Design review of the part shown in the three views and the two pictorial views. Dimensions are in mm from the part's minimum x, y and z. A direction names the side the tool comes from. Coordinates: 2 decimals unless noted, no trailing zeros. Order: outer loops, then holes, each group sorted by start corner. A loop starts at its lowest first (then second) coordinate and runs counter-clockwise, first axis right, second up. Notation, with made-up numbers: (28.5, -4) - (85.5, -4) arc R15 cw to (85.5, 23) - close; hole circle Ø9 at (35.5, 69.25). An arc over 180 degrees is marked (long way). One line per item, written item: value. Start each with the question number.
(1) Mouldability with a two-part tool opening along X and no side actions: class the marked faces 1, 2 and 3 as released by +X, released by -X, zero draft, split by the parting line, or undercut.
(2) Consider section A-A on y = 35. Write out the cut boundary in (x, z).
(3) To check wall thickness, follow line 1 along X through (y, z) = (48.5, 45); line 2 along Z through (x, y) = (4.5, 8.5); line 3 along Y through (x, z) = (46.5, 34). State the ranges of each line that lie inside material, in increasing order.
(4) Consider section D-D on z = 37. Write out the cut boundary in (x, y).
(5) Consider section C-C on z = 9.5. Write out the cut boundary in (x, y).
(6) Consider section B-B on x = 71. Write out the cut boundary in (y, z), then the cut area to 3 significant figures.
(7) For the marked faces 4, 5 and 6, list the 3-axis set-ups (+Z, -Z, +X, -X, +Y, -Y) from which the entire face can be reached by the end or side of a thin tool; tool diameter is ignored.
(8) Clearance check with flat-ended pins moving along their axes: pin 1 (1.5 mm diameter, centred on x = 49.5, z = 38.5, fed in from -Y); pin 2 (12.5 mm diameter, centred on x = 64, y = 44.5, fed in from +Z). State where each tip first meets the part, or that it passes through.
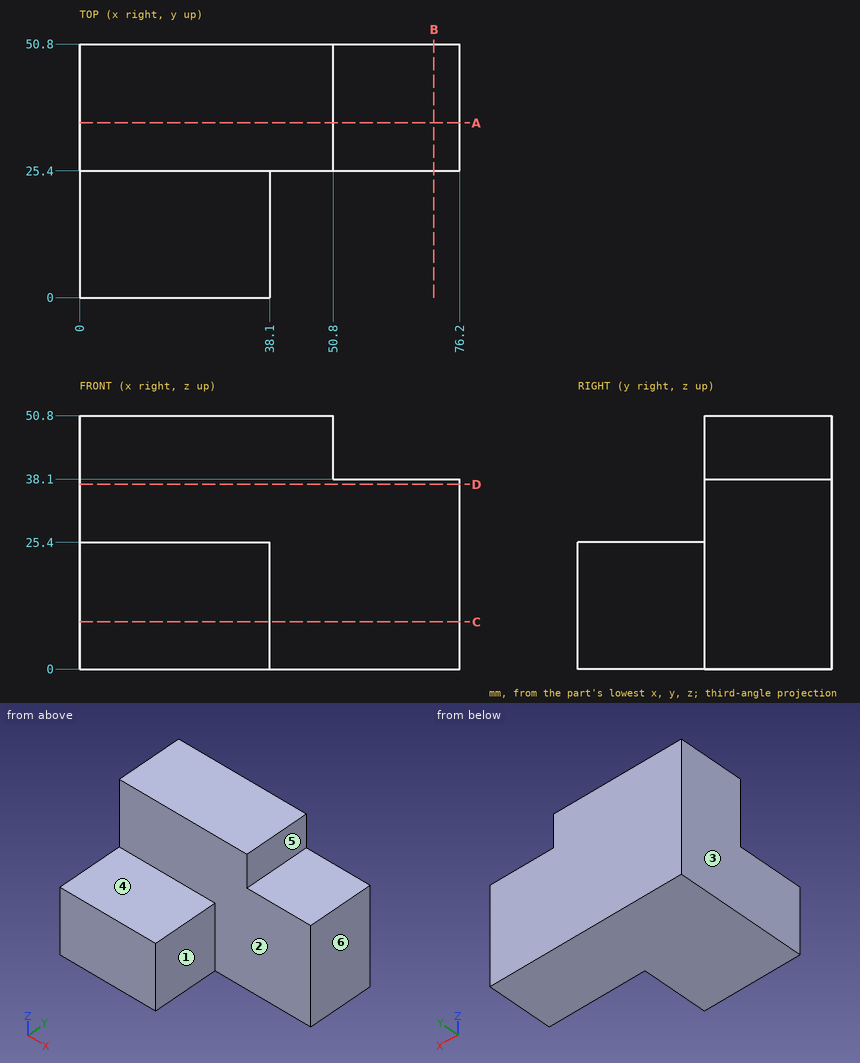
Geometry check:
1. face 1: released by +X
1. face 2: zero draft
1. face 3: released by -X
2. outline: (0, 0) - (76.2, 0) - (76.2, 38.1) - (50.8, 38.1) - (50.8, 50.8) - (0, 50.8) - close
3. line 1: x = 0 to 50.8
3. line 2: z = 0 to 25.4
3. line 3: y = 25.4 to 50.8
4. outline: (0, 25.4) - (76.2, 25.4) - (76.2, 50.8) - (0, 50.8) - close
5. outline: (0, 0) - (38.1, 0) - (38.1, 25.4) - (76.2, 25.4) - (76.2, 50.8) - (0, 50.8) - close
6. outline: (25.4, 0) - (50.8, 0) - (50.8, 38.1) - (25.4, 38.1) - close
6. area: 968 mm^2
7. face 4: +Z, +X, -X, -Y
7. face 5: +Z, +X, +Y, -Y
7. face 6: +Z, -Z, +X, +Y, -Y
8. pin 1: stops at y = 25.4
8. pin 2: stops at z = 38.1
